```python
from build123d import *

# Parameters (mm, degrees)
ESQUISSE1_W             = 70
ESQUISSE1_H             = 54
BOSS_EXTRU_1_DEPTH      = 1
ESQUISSE2_R             = 8.25
ENL_V_MAT_EXTRU_1_DEPTH = 10
ESQUISSE4_R             = 8.25
ENL_V_MAT_EXTRU_3_DEPTH = 10
M3_CLEARANCE_HOLE1_D    = 3.4


with BuildPart() as part:
    # Esquisse1 → Boss.-Extru.1 (new body)
    with BuildSketch(Plane(origin=(0, 0, 0), x_dir=(1, 0, 0), z_dir=(0, 1, 0))):
        Rectangle(ESQUISSE1_W, ESQUISSE1_H)
    extrude(amount=BOSS_EXTRU_1_DEPTH)

    # Esquisse2 → Enlèv. mat.-Extru.1 (cut)
    with BuildSketch(Plane(origin=(0, 1, 0), x_dir=(1, 0, 0), z_dir=(0, 1, 0))):
        with Locations(Location((-14.5, 0, 0), (0, 0, 270))):
            Circle(ESQUISSE2_R)
    extrude(amount=-ENL_V_MAT_EXTRU_1_DEPTH, mode=Mode.SUBTRACT)

    # Esquisse4 → Enlèv. mat.-Extru.3 (cut)
    with BuildSketch(Plane(origin=(0, 1, 0), x_dir=(1, 0, 0), z_dir=(0, 1, 0))):
        with Locations(Location((14.5, 0, 0), (0, 0, 270))):
            Circle(ESQUISSE4_R)
    extrude(amount=-ENL_V_MAT_EXTRU_3_DEPTH, mode=Mode.SUBTRACT)

    # M3 Clearance Hole1 (through all)
    with Locations(Plane(origin=(0, 1, 0), x_dir=(1, 0, 0), z_dir=(0, 1, 0))):
        with Locations((-25, -23), (25, -23), (25, 23), (-25, 23)):
            Hole(M3_CLEARANCE_HOLE1_D / 2)


solid = part.part
```
The model under review builds one solid part; all positions refer to its coordinate system, in mm. Coordinates: 2 decimals unless noted, no trailing zeros. Order: outer loops, then holes, each group sorted by start corner. A loop starts at its lowest first (then second) coordinate and runs counter-clockwise, first axis right, second up. Notation, with made-up numbers: (71.5, 8.5) -> (75.5, 8.5) arc R11 ccw to (75.5, 23.5) -> close; hole circle Ø2 at (-15.5, 25). An arc over 180 degrees is marked (long way). Answer in a Markdown table with one row per item. Add a question column.
Item 1: We need section A-A on x = 14.5. Write out the cut boundary in (y, z).
Item 2: Mouldability with a two-part tool opening along X and no side actions: class faces 1 (the flat face through (0, 0, 0)), 2 (the cylindrical face through (-26.57, 0.49, 23.65)), 3 (the cylindrical face through (23.43, 0.49, 23.65)) as +X half, -X half, draft (parallel to the pull), parting line (faces both ways), or undercut.
Item 3: We need section C-C on z = -1. Write out the cut boundary in (x, y), plus the area to 3 significant figures.
Item 4: We need section D-D on x = -25. Write out the cut boundary in (y, z).
Item 5: To check wall thickness, follow probe 1 along Z at (x, y) = (-25, 0.65); probe 2 along X at (y, z) = (0.4, 0); probe 3 along X at (y, z) = (0.4, 23). State the ranges of each line that lie inside material, in increasing order.
Item 6: We need section B-B on y = 0.7. Write out the cut boundary in (x, z), plus the area to 3 significant figures.
Final values:
| question | item | result |
|---|---|---|
| 1 | outline | (0, -27) -> (1, -27) -> (1, -8.25) -> (0, -8.25) -> close; (0, 8.25) -> (1, 8.25) -> (1, 27) -> (0, 27) -> close |
| 2 | face 1 | draft |
| 2 | face 2 | undercut |
| 2 | face 3 | undercut |
| 3 | outline | (-35, 0) -> (-22.69, 0) -> (-22.69, 1) -> (-35, 1) -> close; (-6.31, 0) -> (6.31, 0) -> (6.31, 1) -> (-6.31, 1) -> close; (22.69, 0) -> (35, 0) -> (35, 1) -> (22.69, 1) -> close |
| 3 | area | 37.2 mm2 |
| 4 | outline | (0, -27) -> (1, -27) -> (1, -24.7) -> (0, -24.7) -> close; (0, -21.3) -> (1, -21.3) -> (1, 21.3) -> (0, 21.3) -> close; (0, 24.7) -> (1, 24.7) -> (1, 27) -> (0, 27) -> close |
| 5 | probe 1 | z = -27 to -24.7, -21.3 to 21.3, 24.7 to 27 |
| 5 | probe 2 | x = -35 to -22.75, -6.25 to 6.25, 22.75 to 35 |
| 5 | probe 3 | x = -35 to -26.7, -23.3 to 23.3, 26.7 to 35 |
| 6 | outline | (-35, -27) -> (35, -27) -> (35, 27) -> (-35, 27) -> close; hole circle Ø3.4 at (-25, -23); hole circle Ø3.4 at (-25, 23); hole circle Ø16.5 at (-14.5, 0); hole circle Ø16.5 at (14.5, 0); hole circle Ø3.4 at (25, -23); hole circle Ø3.4 at (25, 23) |
| 6 | area | 3,320 mm2 |
